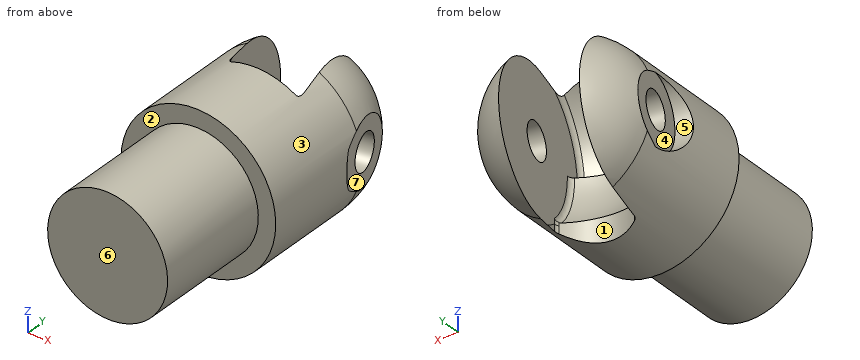
```python
from build123d import *

# Parameters (mm, degrees)
SKETCH1_R                     = 12.9921
BOSS_EXTRUDE1_DEPTH           = 25.4
CUT_EXTRUDE1_DEPTH            = 104.344307451
CUT_EXTRUDE1_DEPTH_BACK       = 104.344307451
SKETCH3_R                     = 3.81
CUT_REVOLVE10_ANGLE           = 90
CUT_REVOLVE10_OTHER_WAY_ANGLE = 180
CUT_EXTRUDE4_DEPTH            = 32.004
FILLET1_R                     = 1.27
SKETCH15_R                    = 7.62
CUT_EXTRUDE5_DEPTH            = 10.16


with BuildPart() as part:
    # Sketch1 → Boss-Extrude1 (new body)
    with BuildSketch(Plane(origin=(0, 0, 0), x_dir=(1, 0, 0), z_dir=(0, 1, 0))):
        with Locations(Location((0, 0, 0), (0, 0, 270))):
            Circle(SKETCH1_R)
    extrude(amount=BOSS_EXTRUDE1_DEPTH)

    # Sketch2 → Revolve1 (revolve)
    with BuildSketch(Plane(origin=(0, 0, 0), x_dir=(0, 0, -1), z_dir=(1, 0, 0))):
        with BuildLine():
            Line((-16.764, 25.4), (-16.764, 49.53))
            ThreePointArc((-16.764, 49.53), (-11.85393808, 61.38393808), (0, 66.294))
            Line((0, 66.294), (0, 25.4))
            Line((0, 25.4), (-16.764, 25.4))
        make_face()
    revolve(axis=Axis((0, 25.4, 0), (0, 1, 0)))

    # Sketch3 → Cut-Extrude1 (cut, two sides: drawn at the far end of the back side and taken through both)
    with BuildSketch(Plane(origin=(-10.366451402, 98.300319395, 0), x_dir=(0, 0, -1), z_dir=(-0.9781476007338062, -0.20791169081775643, 0)).offset(-CUT_EXTRUDE1_DEPTH_BACK)):
        with Locations(Location((0, 49.859877342, 0), (0, 0, 65.612599739))):
            Circle(SKETCH3_R)
    extrude(amount=CUT_EXTRUDE1_DEPTH + CUT_EXTRUDE1_DEPTH_BACK, mode=Mode.SUBTRACT)

    # Sketch11 → Cut-Revolve10 (revolve, cut)
    with BuildSketch(Plane.XY):
        with BuildLine():
            Line((-7.701934208, 47.892903347), (-11.162976054, 64.175825024))
            ThreePointArc((-11.162976054, 64.175825024), (-4.101170935, 67.482510185), (3.695979409, 67.570287171))
            Line((3.695979409, 67.570287171), (7.205035227, 51.061477515))
            Line((7.205035227, 51.061477515), (-7.701934208, 47.892903347))
        make_face()
    revolve(axis=Axis((17.487516564, 53.247086393, 0), (-0.9781476007338064, -0.2079116908177564, 0)), revolution_arc=CUT_REVOLVE10_ANGLE, mode=Mode.SUBTRACT)

    # Sketch11 → Cut-Revolve10 other way (revolve, cut)
    with BuildSketch(Plane.XY):
        with BuildLine():
            Line((-7.701934208, 47.892903347), (-11.162976054, 64.175825024))
            ThreePointArc((-11.162976054, 64.175825024), (-4.101170935, 67.482510185), (3.695979409, 67.570287171))
            Line((3.695979409, 67.570287171), (7.205035227, 51.061477515))
            Line((7.205035227, 51.061477515), (-7.701934208, 47.892903347))
        make_face()
    revolve(axis=Axis((17.487516564, 53.247086393, 0), (0.9781476007338064, 0.2079116908177564, 0)), revolution_arc=CUT_REVOLVE10_OTHER_WAY_ANGLE, mode=Mode.SUBTRACT)

    # Sketch13 → Cut-Revolve11 (revolve, cut)
    with BuildSketch(Plane.XY):
        with BuildLine():
            Line((-8.49407775, 51.619645705), (6.412891685, 54.788219873))
            Line((6.412891685, 54.788219873), (2.927360083, 71.186356794))
            ThreePointArc((2.927360083, 71.186356794), (-4.869286819, 71.216520857), (-11.979609352, 68.017782626))
            Line((-11.979609352, 68.017782626), (-8.49407775, 51.619645705))
        make_face()
    revolve(axis=Axis((-8.49407775, 51.619645705, 0), (0.9781476007338064, 0.20791169081775637, 0)), mode=Mode.SUBTRACT)

    # Sketch14 → Cut-Extrude4 (cut)
    with BuildSketch(Plane.XY):
        with BuildLine():
            Line((-7.701934208, 47.892903347), (-6.149656223, 40.590009601))
            ThreePointArc((-6.149656223, 40.590009601), (1.969552427, 39.042311826), (8.757313212, 43.758583769))
            Line((8.757313212, 43.758583769), (7.205035227, 51.061477515))
            Line((7.205035227, 51.061477515), (-7.701934208, 47.892903347))
        make_face()
    extrude(amount=-CUT_EXTRUDE4_DEPTH, mode=Mode.SUBTRACT)

    # Fillet1
    fillet1_edges = [part.edges().sort_by_distance(p)[0] for p in [
        (10.298585015, 36.507470038, 7.966497668),
        (-4.840027967, 34.428693074, 9.361457334),
        (-5.306564153, 36.623573262, -6.782727573),
        (9.600405282, 39.79214743, -6.782727573),
        (-6.149656223, 40.590009601, -14.000445211),
        (8.757313212, 43.758583769, -13.350191985),
    ]]
    fillet(fillet1_edges, radius=FILLET1_R)

    # Sketch15 → Cut-Extrude5 (cut)
    with BuildSketch(Plane(origin=(-4.834136469, -1.027527427, 0), x_dir=(0, 0, -1), z_dir=(-0.9781476007338062, -0.20791169081775643, 0))):
        with Locations((0, -48.447650664)):
            Circle(SKETCH15_R)
    cut_extrude5 = extrude(amount=CUT_EXTRUDE5_DEPTH, mode=Mode.SUBTRACT)

    # Mirror1: Cut-Extrude5 across plane
    add(cut_extrude5.mirror(Plane(origin=(10.072832966, 2.141046741, 0), x_dir=(0, 0, 1), z_dir=(-0.9781476007338062, -0.20791169081775643, 0))), mode=Mode.SUBTRACT)


solid = part.part
```
The listing builds one solid part. Answer for the finished solid, in the listing's coordinates (mm). Face numbers are marked on the shaded views. A direction names the side the tool comes from. Round coordinates to 2 decimals unless told otherwise and drop trailing zeros. Order: outer loops, then holes, each group sorted by start corner. A loop starts at its lowest first (then second) coordinate and runs counter-clockwise, first axis right, second up. Notation, with made-up numbers: (68, -16.5) - (82, -16.5) arc R16 cw to (82, 11.5) - close; hole circle Ø11 at (-23, -10). An arc over 180 degrees is marked (long way). Put each result on its own line as item: value. Start each with the question number.
(1) Find section A-A (x = 5). Give the vertices of the cut face in (y, z), plus the area to 3 significant figures.
(2) Find section B-B (y = 30). Give the vertices of the cut face in (x, z).
(3) Find section C-C (x = -1.5). Give the vertices of the cut face in (y, z), plus the area to 3 significant figures.
(4) For the marked faces 1, 2, 3 and 4, determine the directions among +Z, -Z, +X, -X, +Y, -Y from which every point of the face is accessible in a straight line to the end or side of a thin tool.
(5) Determine the mould class of the marked faces 5, 6 and 7 for opening direction Y: released by +Y, released by -Y, zero draft, split by the parting line, or undercut.
(6) Find section D-D (z = 1). State how many separate pieces and enclosed holes the cut face has, plus the area to 3 significant figures.
(7) Given P1, Ø8, axis at x = 8, z = 1, coming from the -Y side; P2, Ø1.5, axis at y = 42, z = -12.5, coming from the -X side; P3, Ø5, axis at x = -2, y = 16, coming from the -Z side; P4, Ø1.5, axis at x = -13, z = -3, coming from the +Y side, each flat-ended and moving along its own axis, determine where each tip first touches the part or whether it passes through.
(8) Straight lines are drawn through the part: probe 1 along Z at (x, y) = (14.5, 49.5); probe 2 along Y at (x, z) = (-11.5, -1.5); probe 3 along X at (y, z) = (47, 11.5). For each, find the intervals that lie inside material, in ascending order. Write a range as from..to.
Reply:
1. outline: (0, -11.99) - (25.4, -11.99) - (25.4, -16) - (40.19, -16) - (40.19, -11.54) arc R17.4 cw to (35.81, 0) - (31.81, 0) arc R17.72 cw to (41.91, 16) - (25.4, 16) - (25.4, 11.99) - (0, 11.99) - close; (61.44, -10.69) arc R16 ccw to (61.44, 10.69) - close
1. area: 1,020 mm^2
2. outline: circle Ø33.53 at (0, 0)
3. outline: (0, -12.91) - (25.4, -12.91) - (25.4, -16.7) - (38.88, -16.7) - (38.88, -11.57) arc R18.41 cw to (34.79, 0) - (31.18, 0) arc R18.35 cw to (41.91, 16.7) - (25.4, 16.7) - (25.4, 12.91) - (0, 12.91) - close
3. area: 995 mm^2
4. face 1: -Z
4. face 2: -Y
4. face 3: +Y, -Y
4. face 4: -X
5. face 5: undercut
5. face 6: released by -Y
5. face 7: released by +Y
6. separate pieces: 3
6. enclosed holes: 0
6. area: 1,230 mm^2
7. P1: y = 0
7. P2: x = -11.96
7. P3: z = -12.99
7. P4: y = 60.6
8. probe 1: -8.41..-2.29, 2.29..8.41
8. probe 2: 0..43.51, 50.67..61.64
8. probe 3: -12.2..-7.51, 8.07..12.2
